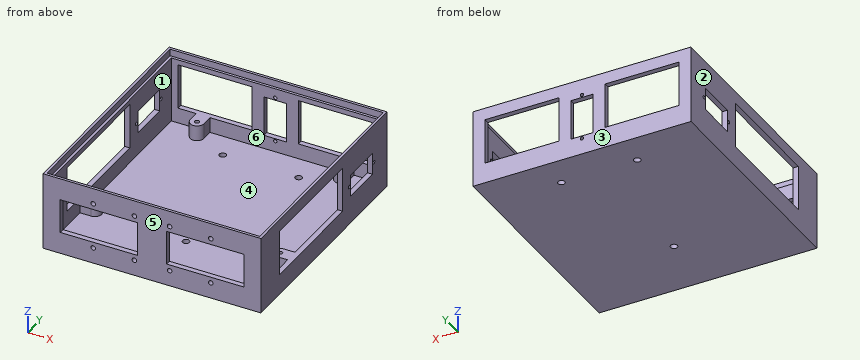
```python
from build123d import *

# Parameters (mm, degrees)
SKETCH1_W           = 127
SKETCH1_H           = 135
BOSS_EXTRUDE1_DEPTH = 45.5
SKETCH2_W           = 121
SKETCH2_H           = 129
CUT_EXTRUDE1_DEPTH  = 42.5
SKETCH2_3_W         = 124
SKETCH2_3_H         = 132
SKETCH2_3_W_2       = 121
SKETCH2_3_H_2       = 129
CUT_EXTRUDE2_DEPTH  = 4
SKETCH3_R           = 1.35
BOSS_EXTRUDE2_DEPTH = 9
SKETCH4_R           = 1.35
BOSS_EXTRUDE3_DEPTH = 9
SKETCH5_R           = 1
SKETCH5_W           = 13
SKETCH5_H           = 23.5
CUT_EXTRUDE5_DEPTH  = 3
SKETCH7_R           = 1
SKETCH7_W           = 13
SKETCH7_H           = 23.5
CUT_EXTRUDE6_DEPTH  = 124
SKETCH8_R           = 1.35
SKETCH8_W           = 45
SKETCH8_H           = 20
CUT_EXTRUDE7_DEPTH  = 3
SKETCH9_R           = 2
CUT_EXTRUDE8_DEPTH  = 3
CUT_EXTRUDE9_REACH  = 152.849
SKETCH10_W          = 26.5
SKETCH10_H          = 67.5
SKETCH11_W          = 43
SKETCH11_H          = 26.5
CUT_EXTRUDE10_DEPTH = 3


with BuildPart() as part:
    # Sketch1 → Boss-Extrude1 (new body)
    with BuildSketch(Plane.XY):
        Rectangle(SKETCH1_W, SKETCH1_H)
    extrude(amount=BOSS_EXTRUDE1_DEPTH)

    # Sketch2 → Cut-Extrude1 (cut)
    with BuildSketch(Plane.XY.offset(45.5)):
        Rectangle(SKETCH2_W, SKETCH2_H)
    extrude(amount=-CUT_EXTRUDE1_DEPTH, mode=Mode.SUBTRACT)

    # Sketch2<3> → Cut-Extrude2 (cut)
    with BuildSketch(Plane.XY.offset(45.5)):
        Rectangle(SKETCH2_3_W, SKETCH2_3_H)
        Rectangle(SKETCH2_3_W_2, SKETCH2_3_H_2, mode=Mode.SUBTRACT)
    extrude(amount=-CUT_EXTRUDE2_DEPTH, mode=Mode.SUBTRACT)

    # Sketch3 → Boss-Extrude2 (add)
    with BuildSketch(Plane.XY.offset(3)):
        with BuildLine():
            Line((38, 64.5), (38, 58))
            ThreePointArc((38, 58), (42, 54), (46, 58))
            Line((46, 58), (46, 64.5))
            Line((46, 64.5), (38, 64.5))
        make_face()
        with Locations((42, 58)):
            Circle(SKETCH3_R, mode=Mode.SUBTRACT)
    boss_extrude2 = extrude(amount=BOSS_EXTRUDE2_DEPTH)

    # Mirror1: Boss-Extrude2 across plane
    add(boss_extrude2.mirror(Plane(origin=(0, 0, 0), x_dir=(0, 0, 1), z_dir=(1, 0, 0))))

    # Sketch4 → Boss-Extrude3 (add)
    with BuildSketch(Plane.XY.offset(3)):
        with BuildLine():
            Line((60.5, -25.4), (54, -25.4))
            ThreePointArc((54, -25.4), (50, -29.4), (54, -33.4))
            Line((54, -33.4), (60.5, -33.4))
            Line((60.5, -33.4), (60.5, -25.4))
        make_face()
        with Locations((54, -29.4)):
            Circle(SKETCH4_R, mode=Mode.SUBTRACT)
    boss_extrude3 = extrude(amount=BOSS_EXTRUDE3_DEPTH)

    # Mirror2: Boss-Extrude3 across plane
    add(boss_extrude3.mirror(Plane(origin=(0, 0, 0), x_dir=(0, 0, 1), z_dir=(1, 0, 0))))

    # Sketch5 → Cut-Extrude5 (cut)
    with BuildSketch(Plane(origin=(0, 67.5, 0), x_dir=(1, 0, 0), z_dir=(0, 1, 0))):
        with Locations(Location((0, -9.5, 0), (0, 0, 180))):
            Circle(SKETCH5_R)
        with Locations(Location((0, -36, 0), (0, 0, 270))):
            Circle(SKETCH5_R)
        with Locations((0, -22.75)):
            Rectangle(SKETCH5_W, SKETCH5_H)
    extrude(amount=-CUT_EXTRUDE5_DEPTH, mode=Mode.SUBTRACT)

    # Sketch7 → Cut-Extrude6 (cut)
    with BuildSketch(Plane(origin=(63.5, 0, 0), x_dir=(0, 0, -1), z_dir=(1, 0, 0))):
        with Locations(Location((-22.75, 53.5, 0), (0, 0, 90))):
            Circle(SKETCH7_R)
        with Locations(Location((-22.75, 27, 0), (0, 0, 90))):
            Circle(SKETCH7_R)
        with Locations((-22.75, 40.25)):
            Rectangle(SKETCH7_W, SKETCH7_H)
    cut_extrude6 = extrude(amount=-CUT_EXTRUDE6_DEPTH, mode=Mode.SUBTRACT)

    # Mirror4: Cut-Extrude6 across plane
    add(cut_extrude6.mirror(Plane(origin=(0, 0, 0), x_dir=(0, 0, 1), z_dir=(1, 0, 0))), mode=Mode.SUBTRACT)

    # Sketch8 → Cut-Extrude7 (cut)
    with BuildSketch(Plane.XZ.offset(67.5)):
        with Locations((-10.25, 36.25)):
            Circle(SKETCH8_R)
        with Locations((-34.25, 36.25)):
            Circle(SKETCH8_R)
        with Locations((-34.25, 9.25)):
            Circle(SKETCH8_R)
        with Locations((-10.25, 9.25)):
            Circle(SKETCH8_R)
        with Locations((-31, 22.75)):
            Rectangle(SKETCH8_W, SKETCH8_H)
    cut_extrude7 = extrude(amount=-CUT_EXTRUDE7_DEPTH, mode=Mode.SUBTRACT)

    # Mirror5: Cut-Extrude7 across plane
    add(cut_extrude7.mirror(Plane(origin=(0, 0, 0), x_dir=(0, 0, 1), z_dir=(1, 0, 0))), mode=Mode.SUBTRACT)

    # Sketch9 → Cut-Extrude8 (cut)
    with BuildSketch(Plane(origin=(0, 0, 0), x_dir=(-1, 0, 0), z_dir=(0, 0, -1))):
        with Locations((-22.1, 48.945)):
            Circle(SKETCH9_R)
        with Locations((0, -31.065)):
            Circle(SKETCH9_R)
    cut_extrude8 = extrude(amount=-CUT_EXTRUDE8_DEPTH, mode=Mode.SUBTRACT)

    # Mirror6: Cut-Extrude8 across plane
    add(cut_extrude8.mirror(Plane(origin=(0, 0, 0), x_dir=(0, 0, 1), z_dir=(1, 0, 0))), mode=Mode.SUBTRACT)

    # Cut-Extrude9: up to this face of the body (flat: up to its plane)
    cut_extrude9_end = Plane(part.part.faces().sort_by_distance((-63.5, -2.152269371, 22.75))[0])
    # Sketch10 → Cut-Extrude9 (cut, up to the picked face)
    with BuildSketch(Plane(origin=(63.5, 0, 0), x_dir=(0, 0, -1), z_dir=(1, 0, 0)), mode=Mode.PRIVATE) as cut_extrude9_sk1:
        with Locations((-25.25, -13.75)):
            Rectangle(SKETCH10_W, SKETCH10_H)
    cut_extrude9_tool1 = split(extrude(cut_extrude9_sk1.sketch, amount=-CUT_EXTRUDE9_REACH, mode=Mode.PRIVATE), bisect_by=cut_extrude9_end, keep=Keep.BOTH, mode=Mode.PRIVATE)
    add(cut_extrude9_tool1.solids().sort_by(Axis((63.5, -13.75, 25.25), (-1, 0, 0)))[0], mode=Mode.SUBTRACT)

    # Sketch11 → Cut-Extrude10 (cut)
    with BuildSketch(Plane(origin=(0, 67.5, 0), x_dir=(1, 0, 0), z_dir=(0, 1, 0))):
        with Locations((35, -25.25)):
            Rectangle(SKETCH11_W, SKETCH11_H)
    cut_extrude10 = extrude(amount=-CUT_EXTRUDE10_DEPTH, mode=Mode.SUBTRACT)

    # Mirror7: Cut-Extrude10 across plane
    add(cut_extrude10.mirror(Plane(origin=(0, 0, 0), x_dir=(0, 0, 1), z_dir=(1, 0, 0))), mode=Mode.SUBTRACT)


solid = part.part
```
Here's how the part is built. I have some questions about the finished solid (model axes, mm). Face numbers are marked on the shaded views. A direction names the side the tool comes from. Round coordinates to 2 decimals unless told otherwise and drop trailing zeros. Write each loop counter-clockwise with the first axis right and the second up, starting at its lowest first coordinate (ties: lowest second). Pieces come first, ordered by that corner, then holes.
Q1. If we section it at C-C on y = -16.5: Write out the boundary of the cut face in (x, z).
Q2. If we section it at A-A on x = 30: Write out the boundary of the cut face in (y, z), plus the area to 4 significant figures.
Q3. Please list where these lines run through material, in increasing order: probe 1 along X at (y, z) = (35, 13.5); probe 2 along Y at (x, z) = (41, 43); probe 3 along X at (y, z) = (-29, 8).
Q4. Will these pins go through, and if not, where does the flat tip stop? P1, Ø8, axis at x = 38, z = 34, coming from the +Y side; P2, Ø10, axis at x = -1.5, y = -14, coming from the +Z side; P3, Ø2, axis at x = 54.5, y = -29.5, coming from the +Z side; P4, Ø3.5, axis at x = 0, y = -31.065, coming from the +Z side.
Q5. Which directions (+Z, -Z, +X, -X, +Y, -Y) give clear straight access to the entire face, cutting with the end or side of a thin tool? Please do the marked faces 5 and 6.
Q6. If we section it at B-B on x = -22.1: Write out the boundary of the cut face in (y, z) (3 decimals), plus the area to 4 significant figures.
Q7. If we mould it in two halves opening along X, with no side actions, what happens to the marked faces 1, 2, 3 and 4? For each: +X half, -X half, draft (parallel to the pull), parting line (faces both ways), or undercut.
Answer below:
1. outline: (-63.5, 0) - (63.5, 0) - (63.5, 12) - (60.5, 12) - (60.5, 3) - (-60.5, 3) - (-60.5, 12) - (-63.5, 12) - close; (-63.5, 38.5) - (-60.5, 38.5) - (-60.5, 41.5) - (-62, 41.5) - (-62, 45.5) - (-63.5, 45.5) - close; (60.5, 38.5) - (63.5, 38.5) - (63.5, 45.5) - (62, 45.5) - (62, 41.5) - (60.5, 41.5) - close
2. outline: (-67.5, 0) - (67.5, 0) - (67.5, 12) - (64.5, 12) - (64.5, 3) - (-64.5, 3) - (-64.5, 12.75) - (-67.5, 12.75) - close; (-67.5, 32.75) - (-64.5, 32.75) - (-64.5, 41.5) - (-66, 41.5) - (-66, 45.5) - (-67.5, 45.5) - close; (64.5, 38.5) - (67.5, 38.5) - (67.5, 45.5) - (66, 45.5) - (66, 41.5) - (64.5, 41.5) - close
2. area: 508.5 mm2
3. probe 1: x = -63.5 to -60.5, 60.5 to 63.5
3. probe 2: y = -67.5 to -66, 66 to 67.5
3. probe 3: x = -63.5 to -55.29, -52.71 to -50.02, 50.02 to 52.71, 55.29 to 63.5
4. P1: stops at y = -64.5
4. P2: stops at z = 3
4. P3: stops at z = 12
4. P4: passes through
5. face 5: +Z, -Z, +X, -X, -Y
5. face 6: +Z
6. outline: (-67.5, 0) - (46.945, 0) - (46.945, 3) - (-64.5, 3) - (-64.5, 12.75) - (-67.5, 12.75) - close; (-67.5, 32.75) - (-64.5, 32.75) - (-64.5, 41.5) - (-66, 41.5) - (-66, 45.5) - (-67.5, 45.5) - close; (50.945, 0) - (67.5, 0) - (67.5, 12) - (64.5, 12) - (64.5, 3) - (50.945, 3) - close; (64.5, 38.5) - (67.5, 38.5) - (67.5, 45.5) - (66, 45.5) - (66, 41.5) - (64.5, 41.5) - close
6. area: 496.5 mm2
7. face 1: undercut
7. face 2: -X half
7. face 3: draft
7. face 4: undercut
